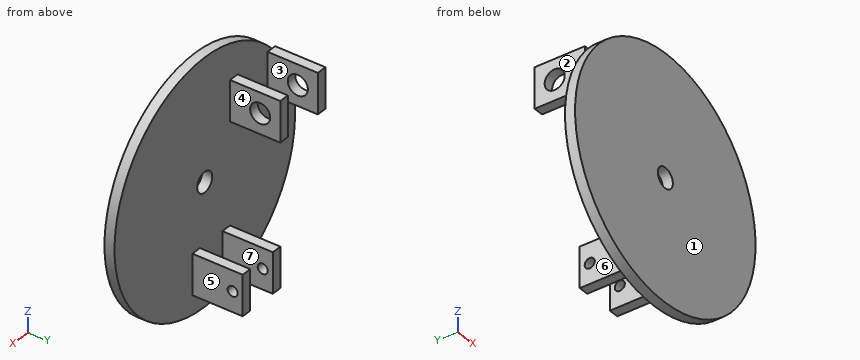
from build123d import *

# Parameters (mm, degrees)
SKETCH1_R           = 76.2
BOSS_EXTRUDE1_DEPTH = 6.35
SKETCH2_R           = 6.35
CUT_EXTRUDE1_DEPTH  = 108.95
SKETCH3_W           = 6.35
SKETCH3_H           = 25.4
BOSS_EXTRUDE2_DEPTH = 31.75
CUT_EXTRUDE2_REACH  = 131.524
SKETCH4_R           = 6.35
SKETCH5_W           = 6.35
SKETCH5_H           = 25.4
BOSS_EXTRUDE3_DEPTH = 31.75
CUT_EXTRUDE3_REACH  = 131.524
SKETCH6_R           = 3.175


with BuildPart() as part:
    # Sketch1 → Boss-Extrude1 (new body)
    with BuildSketch(Plane(origin=(0, 0, 0), x_dir=(1, 0, 0), z_dir=(0, 1, 0))):
        with Locations(Location((0, 0, 0), (0, 0, 270))):
            Circle(SKETCH1_R)
    extrude(amount=BOSS_EXTRUDE1_DEPTH)

    # Sketch2 → Cut-Extrude1 (cut, through all)
    with BuildSketch(Plane.XZ):
        with Locations(Location((0, 0, 0), (0, 0, 270))):
            Circle(SKETCH2_R)
    extrude(amount=-CUT_EXTRUDE1_DEPTH, mode=Mode.SUBTRACT)

    # Sketch3 → Boss-Extrude2 (add)
    with BuildSketch(Plane(origin=(0, 6.35, 0), x_dir=(1, 0, 0), z_dir=(0, 1, 0))):
        with Locations((-56.28767, -38.1)):
            Rectangle(SKETCH3_W, SKETCH3_H)
        with Locations((-24.53767, -38.1)):
            Rectangle(SKETCH3_W, SKETCH3_H)
    extrude(amount=BOSS_EXTRUDE2_DEPTH)

    # Cut-Extrude2: up to this face of the body (flat: up to its plane)
    cut_extrude2_end = Plane(part.part.faces().sort_by_distance((-59.46267, 22.225, 38.1))[0])
    # Sketch4 → Cut-Extrude2 (cut, up to the picked face)
    with BuildSketch(Plane(origin=(-21.36267, 0, 0), x_dir=(0, 0, -1), z_dir=(1, 0, 0)), mode=Mode.PRIVATE) as cut_extrude2_sk1:
        with Locations((-38.1, 25.4)):
            Circle(SKETCH4_R)
    cut_extrude2_tool1 = split(extrude(cut_extrude2_sk1.sketch, amount=-CUT_EXTRUDE2_REACH, mode=Mode.PRIVATE), bisect_by=cut_extrude2_end, keep=Keep.BOTH, mode=Mode.PRIVATE)
    add(cut_extrude2_tool1.solids().sort_by(Axis((-21.36267, 25.4, 38.1), (-1, 0, 0)))[0], mode=Mode.SUBTRACT)

    # Sketch5 → Boss-Extrude3 (add)
    with BuildSketch(Plane(origin=(0, 6.35, 0), x_dir=(1, 0, 0), z_dir=(0, 1, 0))):
        with Locations((-18.18767, 50.8)):
            Rectangle(SKETCH5_W, SKETCH5_H)
        with Locations((7.21233, 50.8)):
            Rectangle(SKETCH5_W, SKETCH5_H)
    extrude(amount=BOSS_EXTRUDE3_DEPTH)

    # Cut-Extrude3: up to this face of the body (flat: up to its plane)
    cut_extrude3_end = Plane(part.part.faces().sort_by_distance((10.38733, 22.225, -50.8))[0])
    # Sketch6 → Cut-Extrude3 (cut, up to the picked face)
    with BuildSketch(Plane.ZY.offset(21.36267), mode=Mode.PRIVATE) as cut_extrude3_sk1:
        with Locations((-50.8, 31.75)):
            Circle(SKETCH6_R)
    cut_extrude3_tool1 = split(extrude(cut_extrude3_sk1.sketch, amount=-CUT_EXTRUDE3_REACH, mode=Mode.PRIVATE), bisect_by=cut_extrude3_end, keep=Keep.BOTH, mode=Mode.PRIVATE)
    add(cut_extrude3_tool1.solids().sort_by(Axis((-21.36267, 31.75, -50.8), (1, 0, 0)))[0], mode=Mode.SUBTRACT)


solid = part.part
Can you work these out from the model? Positions are in its coordinate system, mm. Face numbers are marked on the shaded views. A direction names the side the tool comes from. Give positions to 0.01 mm unless a question says otherwise; leave off trailing zeros. Loops run counter-clockwise (first coordinate to the right, second up) from the corner with the lowest first, then second, coordinate; pieces in that order, holes last. Notation, with made-up numbers: M -9,63 L 5,63 A29 ccw 5,92 Z; hole C -3,39.5 d8. An arc over 180 degrees is marked long. One line per item, written item: value.
1) Imagine slicing it at D-D on y = 25.4. Write out the boundary of the cut face in (x, z).
Geometry check:
outline: M -59.46,25.4 L -53.11,25.4 L -53.11,31.75 L -59.46,31.75 Z; M -59.46,44.45 L -53.11,44.45 L -53.11,50.8 L -59.46,50.8 Z; M -27.71,25.4 L -21.36,25.4 L -21.36,31.75 L -27.71,31.75 Z; M -27.71,44.45 L -21.36,44.45 L -21.36,50.8 L -27.71,50.8 Z; M -21.36,-63.5 L -15.01,-63.5 L -15.01,-38.1 L -21.36,-38.1 Z; M 4.04,-63.5 L 10.39,-63.5 L 10.39,-38.1 L 4.04,-38.1 Z
2) On a 3-axis mill with a long thin cutter (end or side, diameter ignored), from which of +Z, -Z, +X, -X, +Y, -Y can I reach the whole of each face in a straight line? I mean the marked faces 4, 5, 6 and 7. Say none if no direction works.
Geometry check:
face 4: +Z, +X, +Y
face 5: +Z, -Z, +X, +Y
face 6: -Z, -X, +Y
face 7: +Z, -Z, +Y
3) Thinking about a two-plate mould opening in X: for the marked faces 1, 2 and 3, which applies, +X half, -X half, draft (parallel to the pull), parting line (faces both ways), or undercut?
Geometry check:
face 1: draft
face 2: -X half
face 3: undercut
4) Imagine slicing it at C-C on z = 0. Write out the boundary of the cut face in (x, y).
Geometry check:
outline: M -76.2,0 L -6.35,0 L -6.35,6.35 L -76.2,6.35 Z; M 6.35,0 L 76.2,0 L 76.2,6.35 L 6.35,6.35 Z
5) Imagine slicing it at A-A on x = 0. Write out the boundary of the cut face in (y, z), and give its area (3 significant figures).
Geometry check:
outline: M 0,-76.2 L 6.35,-76.2 L 6.35,-6.35 L 0,-6.35 Z; M 0,6.35 L 6.35,6.35 L 6.35,76.2 L 0,76.2 Z
area: 887 mm²
6) I'm going to push flat-ended pins straight in: pin 1 (12.5 mm diameter, centred on y = 21, z = 37.5, fed in from +X); pin 2 (10 mm diameter, centred on y = 31.75, z = -50.8, fed in from +X); pin 3 (12 mm diameter, centred on x = 57.5, y = 6, fed in from -Z). Where does each tip first touch, or does it pass through?
Geometry check:
pin 1: stops at x = -21.36
pin 2: stops at x = 10.39
pin 3: stops at z = -56.16
7) Please list where these lines run through material, in increasing order: line 1 (X direction, y = 25, z = -44); line 2 (Y direction, x = -25, z = 38); line 3 (Y direction, x = -37, z = -16).
Geometry check:
line 1: x = -21.36 to -15.01, 4.04 to 10.39
line 2: y = 0 to 19.05, 31.75 to 38.1
line 3: y = 0 to 6.35
8) Imagine slicing it at B-B on y = 9. Write out the boundary of the cut face in (x, z).
Geometry check:
outline: M -59.46,25.4 L -53.11,25.4 L -53.11,50.8 L -59.46,50.8 Z; M -27.71,25.4 L -21.36,25.4 L -21.36,50.8 L -27.71,50.8 Z; M -21.36,-63.5 L -15.01,-63.5 L -15.01,-38.1 L -21.36,-38.1 Z; M 4.04,-63.5 L 10.39,-63.5 L 10.39,-38.1 L 4.04,-38.1 Z
